Model file for the job. Use its own axes, mm. A direction names the side the tool comes from. Round coordinates to 2 decimals unless told otherwise and drop trailing zeros. Loops run counter-clockwise (first coordinate to the right, second up) from the corner with the lowest first, then second, coordinate; pieces in that order, holes last. Notation, with made-up numbers: (8, 21) -> (22, 21) arc R20 cw to (22, 36) -> close; hole circle Ø2 at (-35.5, 14.25). An arc over 180 degrees is marked (long way). Use a Markdown table: item, result. Add a question column.
```python
from build123d import *

# Parameters (mm, degrees)
SKETCH_R        = 90
SKETCH_R_2      = 1.8
SKETCH_R_3      = 12
PAD_DEPTH       = 5
SKETCH001_R     = 4.25
POCKET_DEPTH    = 3
POCKET001_DEPTH = 3


with BuildPart() as part:
    # Sketch → Pad (new body)
    with BuildSketch(Plane.XY):
        Circle(SKETCH_R)
        with Locations((-40, 69.282032)):
            Circle(SKETCH_R_2, mode=Mode.SUBTRACT)
        with Locations((40, 69.282032)):
            Circle(SKETCH_R_2, mode=Mode.SUBTRACT)
        with Locations((80, 0)):
            Circle(SKETCH_R_2, mode=Mode.SUBTRACT)
        with Locations((40, -69.282032)):
            Circle(SKETCH_R_2, mode=Mode.SUBTRACT)
        with Locations((-40, -69.282032)):
            Circle(SKETCH_R_2, mode=Mode.SUBTRACT)
        with Locations((-80, 0)):
            Circle(SKETCH_R_2, mode=Mode.SUBTRACT)
        Circle(SKETCH_R_3, mode=Mode.SUBTRACT)
        with Locations((-12, 12)):
            Circle(SKETCH_R_2, mode=Mode.SUBTRACT)
        with Locations((12, 12)):
            Circle(SKETCH_R_2, mode=Mode.SUBTRACT)
        with Locations((12, -12)):
            Circle(SKETCH_R_2, mode=Mode.SUBTRACT)
        with Locations((-12, -12)):
            Circle(SKETCH_R_2, mode=Mode.SUBTRACT)
    extrude(amount=PAD_DEPTH)

    # Sketch001 → Pocket (cut)
    with BuildSketch(Plane(origin=(0, 0, 0), x_dir=(1, 0, 0), z_dir=(0, 0, -1))):
        with Locations((-40, 69.282032)):
            Circle(SKETCH001_R)
        with Locations((40, 69.282032)):
            Circle(SKETCH001_R)
        with Locations((80, 0)):
            Circle(SKETCH001_R)
        with Locations((40, -69.282032)):
            Circle(SKETCH001_R)
        with Locations((-40, -69.282032)):
            Circle(SKETCH001_R)
        with Locations((-80, 0)):
            Circle(SKETCH001_R)
    extrude(amount=-POCKET_DEPTH, mode=Mode.SUBTRACT)

    # Sketch002 → Pocket001 (cut)
    with BuildSketch(Plane(origin=(0, 0, 0), x_dir=(1, 0, 0), z_dir=(0, 0, -1))):
        Polygon((-8.845014, 11.219894), (-9.746916, 14.342245), (-12.901902, 15.122351), (-15.154986, 12.780106), (-14.253084, 9.657755), (-11.098098, 8.877649), align=None)
        Polygon((14.253084, 9.657755), (15.154986, 12.780106), (12.901902, 15.122351), (9.746916, 14.342245), (8.845014, 11.219894), (11.098098, 8.877649), align=None)
        Polygon((12.901902, -15.122351), (15.154986, -12.780106), (14.253084, -9.657755), (11.098098, -8.877649), (8.845014, -11.219894), (9.746916, -14.342245), align=None)
        Polygon((-9.746916, -14.342245), (-8.845014, -11.219894), (-11.098098, -8.877649), (-14.253084, -9.657755), (-15.154986, -12.780106), (-12.901902, -15.122351), align=None)
    extrude(amount=-POCKET001_DEPTH, mode=Mode.SUBTRACT)


solid = part.part
```
1) Cut at C-C on x = -56.5. Write the cut outline in (y, z), and give its area (3 significant figures).
2) Tool access for faces 1 (the face through (-1, -19, 5)), 2 (the face through (42, -69, 3)): list every direction of +Z, -Z, +X, -X, +Y, -Y with a clear straight run to the whole face (end or side of a thin tool).
3) Pin check, flat tips, straight feed: pin 1 Ø2 at (y, z) = (49.5, 4) entering from +X; pin 2 Ø2.5 at (x, y) = (-39.5, 67.5) entering from -Z; pin 3 Ø3 at (x, z) = (-40.5, 4.5) entering from +Y. Stop position of each tip, or through.
4) Cut at B-B on z = 4.1. Count the separate pieces of the cut face and the enclosed holes in it, and give its area (3 significant figures).
5) Cut at A-A on x = -1. Write the cut outline in (y, z).
6) Pull direction X, two halves, no side cores. Call faces 3 (the face through (41.53, -79.845, 2.465)), 4 (the face through (-11.99, 0.53, 2.46)), 5 (the face through (-13.45, 13.34, 3)), 6 (the face through (-1, -19, 0)): +X half, -X half, draft (parallel to the pull), parting line (faces both ways), or undercut.
7) Wall check: probe 1 along X at (y, z) = (-11, 2.25); probe 2 along X at (y, z) = (72.5, 1.15); probe 3 along X at (y, z) = (-37.5, 1.8). Give the ranges that are in metal, low to high. Write a range as from..to.
8) Cut at D-D on y = -60. Write the cut outline in (x, z), and give its area (3 significant figures).
Established:
| question | item | result |
|---|---|---|
| 1 | outline | (-70.06, 0) -> (70.06, 0) -> (70.06, 5) -> (-70.06, 5) -> close |
| 1 | area | 701 mm^2 |
| 2 | face 1 | +Z, +X, -X, +Y, -Y |
| 2 | face 2 | -Z |
| 3 | pin 1 | stops at x = 75.81 |
| 3 | pin 2 | stops at z = 3 |
| 3 | pin 3 | stops at y = 81.11 |
| 4 | separate pieces | 1 |
| 4 | enclosed holes | 11 |
| 4 | area | 24,900 mm^2 |
| 5 | outline | (-89.99, 0) -> (-11.96, 0) -> (-11.96, 5) -> (-89.99, 5) -> close; (11.96, 0) -> (89.99, 0) -> (89.99, 5) -> (11.96, 5) -> close |
| 6 | face 3 | parting line |
| 6 | face 4 | undercut |
| 6 | face 5 | undercut |
| 6 | face 6 | draft |
| 7 | probe 1 | x = -89.33..-14.64, -9.06..-4.8, 4.8..9.06, 14.64..89.33 |
| 7 | probe 2 | x = -53.33..-42.78, -37.22..37.22, 42.78..53.33 |
| 7 | probe 3 | x = -81.82..81.82 |
| 8 | outline | (-67.08, 0) -> (67.08, 0) -> (67.08, 5) -> (-67.08, 5) -> close |
| 8 | area | 671 mm^2 |
